Answer from the drawing. Dimensions are ordinates in mm from the lowest x, y and z of the part. A direction names the side the tool comes from. Round coordinates to 2 decimals unless told otherwise and drop trailing zeros. Write each loop counter-clockwise with the first axis right and the second up, starting at its lowest first coordinate (ties: lowest second). Pieces come first, ordered by that corner, then holes. Notation, with made-up numbers: (67, -5) - (114, -5) arc R19 ccw to (114, 4) - close; hole circle Ø2 at (-22, 84). An arc over 180 degrees is marked (long way). Return JSON: item names as keys, results as strings. Group by question number.
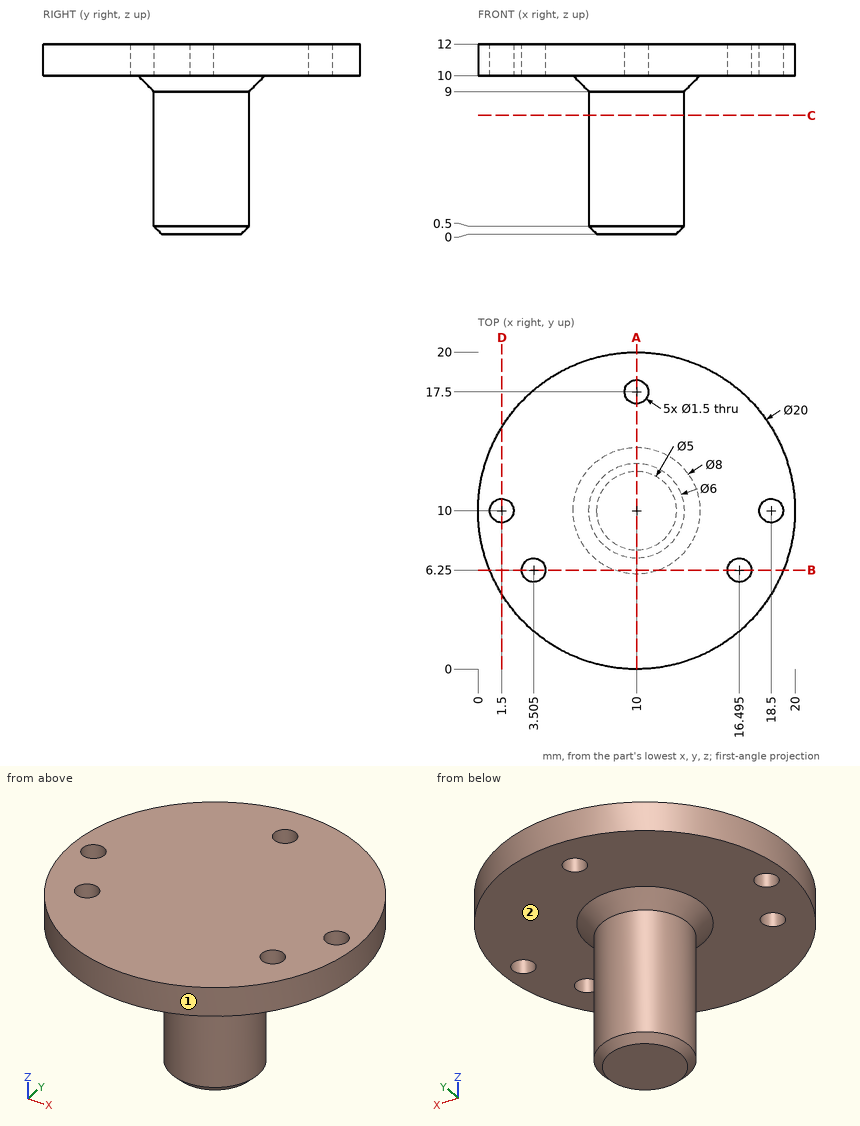
(1) Consider line 1 (Y direction, x = 10, z = 11.1); line 2 (Z direction, x = 17.5, y = 4.25); line 3 (Y direction, x = 7.5, z = 6). Determine where each line is inside the solid, lowest interval first.
(2) Find section A-A (x = 10). Write down the section's boundary in (y, z).
(3) Flat-ended cylindrical pins translate along their axes: pin 1 (5 mm diameter, centred on x = 6, y = 2, fed in from -Z); pin 2 (6 mm diameter, centred on x = 5.5, z = 10.5, fed in from -Y). Find the tip coordinate at first contact, or state that the pin passes through.
(4) Find section B-B (y = 6.25). State how many separate pieces and enclosed holes the cut face has.
(5) Find section D-D (x = 1.5). Write down the section's boundary in (y, z), plus the area to 3 significant figures.
(6) For the marked faces 1 and 2, determine the directions among +Z, -Z, +X, -X, +Y, -Y from which every point of the face is accessible in a straight line to the end or side of a thin tool.
(7) Find section C-C (z = 7.5). Write down the section's boundary in (x, y).
Check sheet entries:
{
 "1": {"line 1": "y = 0 to 16.75, 18.25 to 20", "line 2": "z = 10 to 12", "line 3": "y = 8.34 to 11.66"},
 "2": {"outline": "(0, 10) - (6, 10) - (7, 9) - (7, 0.5) - (7.5, 0) - (12.5, 0) - (13, 0.5) - (13, 9) - (14, 10) - (16.75, 10) - (16.75, 12) - (0, 12) - close; (18.25, 10) - (20, 10) - (20, 12) - (18.25, 12) - close"},
 "3": {"pin 1": "stops at z = 10", "pin 2": "stops at y = 0.11"},
 "4": {"separate pieces": "3", "enclosed holes": "0"},
 "5": {"outline": "(4.73, 10) - (9.25, 10) - (9.25, 12) - (4.73, 12) - close; (10.75, 10) - (15.27, 10) - (15.27, 12) - (10.75, 12) - close", "area": "18.1 mm^2"},
 "6": {"face 1": "+Z, -Z", "face 2": "-Z"},
 "7": {"outline": "circle Ø6 at (10, 10)"}
}
